from build123d import *

# Parameters (mm, degrees)
CONG_1_R = 0.25


with BuildPart() as part:
    # Esquisse1 → Révolution1 (revolve)
    with BuildSketch(Plane.XY):
        with BuildLine():
            Line((0, 0), (-4.5, 0))
            ThreePointArc((-4.5, 0), (-5.914213562, 0.585786438), (-6.5, 2))
            Line((-6.5, 2), (-6.5, 5.2))
            Line((-6.5, 5.2), (-8, 5.2))
            Line((-8, 5.2), (-8, 8.8))
            Line((-8, 8.8), (-3.620773398, 8.8))
            Line((-3.620773398, 8.8), (-3.620773398, 7.8))
            ThreePointArc((-3.620773398, 7.8), (-2.144761059, 9.476388603), (0, 10.1))
            Line((0, 10.1), (0, 0))
        make_face()
    revolve(axis=Axis((0, 10.1, 0), (0, -1, 0)))

    # Congé1
    cong_1_edges = [part.edges().sort_by_distance(p)[0] for p in [
        (8, 8.8, 0),
        (8, 5.2, 0),
    ]]
    fillet(cong_1_edges, radius=CONG_1_R)


solid = part.part
Geometry: final body of the model. Coordinates: model frame, mm. A direction names the side the tool comes from. Give positions to 0.01 mm unless a question says otherwise; leave off trailing zeros. Write each loop counter-clockwise with the first axis right and the second up, starting at its lowest first coordinate (ties: lowest second). Pieces come first, ordered by that corner, then holes. Notation, with made-up numbers: (26, 73) -> (45, 73) arc R21 cw to (45, 78) -> close; hole circle Ø1 at (82, 25). An arc over 180 degrees is marked (long way). Answer as a JSON object with one key per item and string values.
1. Cut plane B-B on y = 8.25. Output: boundary loops of the cut face in (x, z), and give its area (3 significant figures).
Ans:
{"outline": "circle Ø16 at (0, 0); circle Ø6.75 at (0, 0); hole circle Ø7.24 at (0, 0)", "area": "196 mm^2"}
2. Cut plane A-A on z = 0. Output: boundary loops of the cut face in (x, y).
Ans:
{"outline": "(-8, 5.45) arc R0.25 ccw to (-7.75, 5.2) -> (-6.5, 5.2) -> (-6.5, 2) arc R2 ccw to (-4.5, 0) -> (4.5, 0) arc R2 ccw to (6.5, 2) -> (6.5, 5.2) -> (7.75, 5.2) arc R0.25 ccw to (8, 5.45) -> (8, 8.55) arc R0.25 ccw to (7.75, 8.8) -> (3.62, 8.8) -> (3.62, 7.8) arc R4 ccw to (-3.62, 7.8) -> (-3.62, 8.8) -> (-7.75, 8.8) arc R0.25 ccw to (-8, 8.55) -> close"}
3. Access query for faces 4 (the flat face through (-3.34, 8.8, -1.83)), 5 (the cylindrical face through (1.73, 7.02, 7.81)). Directions: +Z, -Z, +X, -X, +Y, -Y. A direction counts if a zero-diameter tool reaches every point of the face in a straight line with its end or side. Return the directions, or none.
Ans:
{"face 4": "+Y", "face 5": "+Y, -Y"}
4. Mould query, pull axis X, two halves, no side actions, for faces 1 (the flat face through (0, 0, 0)), 2 (the cylindrical face through (-3.454, 8.293, -1.088)), 3 (the cylindrical face through (5.158, 3.622, 3.955)). Classes: pulls with the +X half, pulls with the -X half, needs draft (parallel to the pull), parting line crosses it, or undercut.
Ans:
{"face 1": "needs draft", "face 2": "undercut", "face 3": "parting line crosses it"}
5. Ray query, probe 1 along Z at (x, y) = (0, 8.35); probe 2 along X at (y, z) = (8.5, -0.5); probe 3 along X at (y, z) = (8.1, 0). Return the intervals inside material, ascending. Write a range as from..to.
Ans:
{"probe 1": "z = -8..-3.62, -3.31..3.31, 3.62..8", "probe 2": "x = -7.98..-3.59, -3.16..3.16, 3.59..7.98", "probe 3": "x = -8..-3.62, -3.46..3.46, 3.62..8"}
6. Cut plane D-D on y = 3.5. Output: boundary loops of the cut face in (x, z).
Ans:
{"outline": "circle Ø13 at (0, 0)"}
7. Cut plane C-C on x = 0. Output: boundary loops of the cut face in (y, z).
Ans:
{"outline": "(0, -4.5) arc R2 ccw to (2, -6.5) -> (5.2, -6.5) -> (5.2, -7.75) arc R0.25 ccw to (5.45, -8) -> (8.55, -8) arc R0.25 ccw to (8.8, -7.75) -> (8.8, -3.62) -> (7.8, -3.62) arc R4 ccw to (7.8, 3.62) -> (8.8, 3.62) -> (8.8, 7.75) arc R0.25 ccw to (8.55, 8) -> (5.45, 8) arc R0.25 ccw to (5.2, 7.75) -> (5.2, 6.5) -> (2, 6.5) arc R2 ccw to (0, 4.5) -> close"}
8. Contact query for flat-ended pins moving along their axis: pin 1 (1 mm diameter, centred on x = -0.5, z = -2, fed in from +Y); pin 2 (1 mm diameter, centred on x = 2, z = 5.5, fed in from +Y); pin 3 (4.5 mm diameter, centred on x = -2, z = 3, fed in from +Y). Output: stop coordinate, or through.
Ans:
{"pin 1": "stops at y = 9.78", "pin 2": "stops at y = 8.8", "pin 3": "stops at y = 9.86"}
